Model file for the job. Use its own axes, mm. Face numbers are marked on the shaded views. A direction names the side the tool comes from. Round coordinates to 2 decimals unless told otherwise and drop trailing zeros. Order: outer loops, then holes, each group sorted by start corner. A loop starts at its lowest first (then second) coordinate and runs counter-clockwise, first axis right, second up. Notation, with made-up numbers: (76, 17) -> (88, 17) arc R27 cw to (88, 45) -> close; hole circle Ø3 at (-12.5, 58). An arc over 180 degrees is marked (long way). Put each result on its own line as item: value. Start each with the question number.
Q1. Probe L1, parallel to Z at x = -1.55, y = -3.25; L2, parallel to Y at x = 0, z = -4.15; L3, parallel to Z at x = -1.5, y = -1.25. List the from-to ranges inside material, lowest first.
Q2. Pull direction Z, two halves, no side cores. Call the marked faces 3, 4 and 5: released by +Z, released by -Z, zero draft, split by the parting line, or undercut.
Q3. Cut at D-D, the plane y = -4.75. List the corners of the cut face in (x, z), and give its area (3 significant figures).
Q4. Cut at B-B, the plane y = -7.25. List the corners of the cut face in (x, z).
Q5. Cut at A-A, the plane x = 1.5. List the corners of the cut face in (y, z), and give its area (3 significant figures).
Q6. 3-axis set-ups, long thin cutter, end or side, ignore diameter. For the marked faces 1 and 2: which of +Z, -Z, +X, -X, +Y, -Y reach the whole face in a straight line?
Q7. Cut at C-C, the plane x = 0. List the corners of the cut face in (y, z), and give its area (3 significant figures).
from build123d import *

# Parameters (mm, degrees)
ESQUISSE1_W                             = 6
ESQUISSE1_H                             = 7.1
T_LE_DE_BASE_PLI_E1_DEPTH               = 1
T_LE_PLI_E_SUR_AR_TE1_STRIP_W           = 5.4732
T_LE_PLI_E_SUR_AR_TE1_STRIP_H           = 1
T_LE_PLI_E_SUR_AR_TE1_STRIP_CUT_DEPTH   = 6
T_LE_PLI_E_SUR_AR_TE1_STRIP_2_W         = 5.4732
T_LE_PLI_E_SUR_AR_TE1_STRIP_2_H         = 1
T_LE_PLI_E_SUR_AR_TE1_STRIP_CUT_2_DEPTH = 6
T_LE_PLI_E_SUR_AR_TE1_DEPTH             = 6
T_LE_PLI_E_SUR_AR_TE1_BEND_DEPTH        = 6
ESQUISSE12_R                            = 1.7
ENL_V_MAT_EXTRU_1_DEPTH                 = 13.482387592


# Sheet-metal steps are written as plain solids
with BuildPart() as part:
    # Esquisse1 → Tôle de base pliée1 (new body)
    with BuildSketch(Plane(origin=(0, 0, 0), x_dir=(1, 0, 0), z_dir=(0, 1, 0))):
        Rectangle(ESQUISSE1_W, ESQUISSE1_H)
    extrude(amount=-T_LE_DE_BASE_PLI_E1_DEPTH)

    # Tôle pliée sur arête1 strip (across the edge) → Tôle pliée sur arête1 strip cut (cut)
    with BuildSketch(Plane(origin=(3, -1, 3.55), x_dir=(0, 0, -1), z_dir=(-1, 0, 0))):
        with Locations((-2, -0.5)):
            Rectangle(T_LE_PLI_E_SUR_AR_TE1_STRIP_W, T_LE_PLI_E_SUR_AR_TE1_STRIP_H)
    extrude(amount=T_LE_PLI_E_SUR_AR_TE1_STRIP_CUT_DEPTH, mode=Mode.SUBTRACT)

    # Tôle pliée sur arête1 strip 2 (across the edge) → Tôle pliée sur arête1 strip cut 2 (cut)
    with BuildSketch(Plane(origin=(-3, -1, -3.55), x_dir=(0, 0, 1), z_dir=(1, 0, 0))):
        with Locations((-2, -0.5)):
            Rectangle(T_LE_PLI_E_SUR_AR_TE1_STRIP_2_W, T_LE_PLI_E_SUR_AR_TE1_STRIP_2_H)
    extrude(amount=T_LE_PLI_E_SUR_AR_TE1_STRIP_CUT_2_DEPTH, mode=Mode.SUBTRACT)

    # Tôle pliée sur arête1 section (across the edge) → Tôle pliée sur arête1 (add)
    with BuildSketch(Plane(origin=(3, -1, 3.55), x_dir=(0, 0, -1), z_dir=(-1, 0, 0))):
        with BuildLine():
            Line((-1, 0.7366), (-1, 7))
            Line((-1, 7), (0, 7))
            Line((0, 7), (0, 0.7366))
            ThreePointArc((0, 0.7366), (0.215745145, 0.215745145), (0.7366, 0))
            Line((0.7366, 0), (0.7366, -1))
            ThreePointArc((0.7366, -1), (-0.491361636, -0.491361636), (-1, 0.7366))
        make_face()
    extrude(amount=T_LE_PLI_E_SUR_AR_TE1_DEPTH)

    # Tôle pliée sur arête1 section 2 (across the edge) → Tôle pliée sur arête1 bend (add)
    with BuildSketch(Plane(origin=(-3, -1, -3.55), x_dir=(0, 0, 1), z_dir=(1, 0, 0))):
        with BuildLine():
            Line((-1, 0.7366), (-1, 7))
            Line((-1, 7), (0, 7))
            Line((0, 7), (0, 0.7366))
            ThreePointArc((0, 0.7366), (0.215745145, 0.215745145), (0.7366, 0))
            Line((0.7366, 0), (0.7366, -1))
            ThreePointArc((0.7366, -1), (-0.491361636, -0.491361636), (-1, 0.7366))
        make_face()
    extrude(amount=T_LE_PLI_E_SUR_AR_TE1_BEND_DEPTH)

    # Esquisse12 → Enlèv. mat.-Extru.1 (cut, through all)
    with BuildSketch(Plane.XY.offset(4.55)):
        with Locations((0, -5)):
            Circle(ESQUISSE12_R)
    extrude(amount=-ENL_V_MAT_EXTRU_1_DEPTH, mode=Mode.SUBTRACT)


solid = part.part
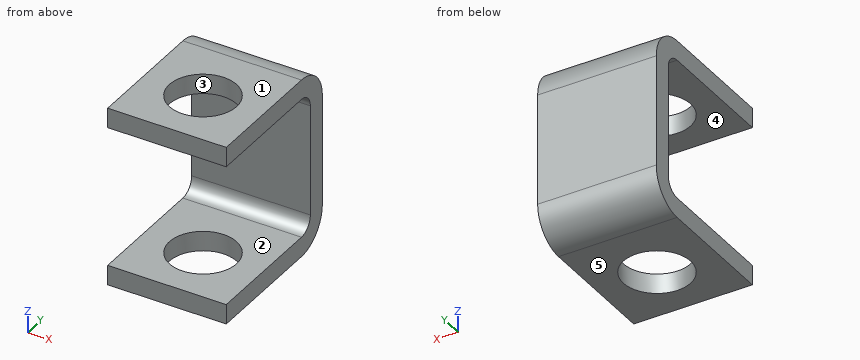
Ans:
1. L1: z = -4.55 to -3.55, 3.55 to 4.55
1. L2: y = -8 to -6.7, -3.3 to -0.63
1. L3: z = -4.48 to -3.37, 3.37 to 4.48
2. face 3: zero draft
2. face 4: undercut
2. face 5: released by -Z
3. outline: (-3, -4.55) -> (-1.68, -4.55) -> (-1.68, -3.55) -> (-3, -3.55) -> close; (-3, 3.55) -> (-1.68, 3.55) -> (-1.68, 4.55) -> (-3, 4.55) -> close; (1.68, -4.55) -> (3, -4.55) -> (3, -3.55) -> (1.68, -3.55) -> close; (1.68, 3.55) -> (3, 3.55) -> (3, 4.55) -> (1.68, 4.55) -> close
3. area: 5.27 mm^2
4. outline: (-3, -4.55) -> (3, -4.55) -> (3, -3.55) -> (-3, -3.55) -> close; (-3, 3.55) -> (3, 3.55) -> (3, 4.55) -> (-3, 4.55) -> close
5. outline: (-8, -4.55) -> (-5.8, -4.55) -> (-5.8, -3.55) -> (-8, -3.55) -> close; (-8, 3.55) -> (-5.8, 3.55) -> (-5.8, 4.55) -> (-8, 4.55) -> close; (-4.2, -4.55) -> (-1.74, -4.55) arc R1.74 ccw to (0, -2.81) -> (0, 2.81) arc R1.74 ccw to (-1.74, 4.55) -> (-4.2, 4.55) -> (-4.2, 3.55) -> (-1.74, 3.55) arc R0.74 cw to (-1, 2.81) -> (-1, -2.81) arc R0.74 cw to (-1.74, -3.55) -> (-4.2, -3.55) -> close
5. area: 18.8 mm^2
6. face 1: +Z, +X, -X, +Y, -Y
6. face 2: +X, -X, -Y
7. outline: (-8, -4.55) -> (-6.7, -4.55) -> (-6.7, -3.55) -> (-8, -3.55) -> close; (-8, 3.55) -> (-6.7, 3.55) -> (-6.7, 4.55) -> (-8, 4.55) -> close; (-3.3, -4.55) -> (-1.74, -4.55) arc R1.74 ccw to (0, -2.81) -> (0, 2.81) arc R1.74 ccw to (-1.74, 4.55) -> (-3.3, 4.55) -> (-3.3, 3.55) -> (-1.74, 3.55) arc R0.74 cw to (-1, 2.81) -> (-1, -2.81) arc R0.74 cw to (-1.74, -3.55) -> (-3.3, -3.55) -> close
7. area: 15.2 mm^2
